Could you check a few things on this drawing? It's one solid part, dimensions in mm from its lowest x, y, z. Give positions to 0.01 mm unless a question says otherwise; leave off trailing zeros. Order: outer loops, then holes, each group sorted by start corner. A loop starts at its lowest first (then second) coordinate and runs counter-clockwise, first axis right, second up.
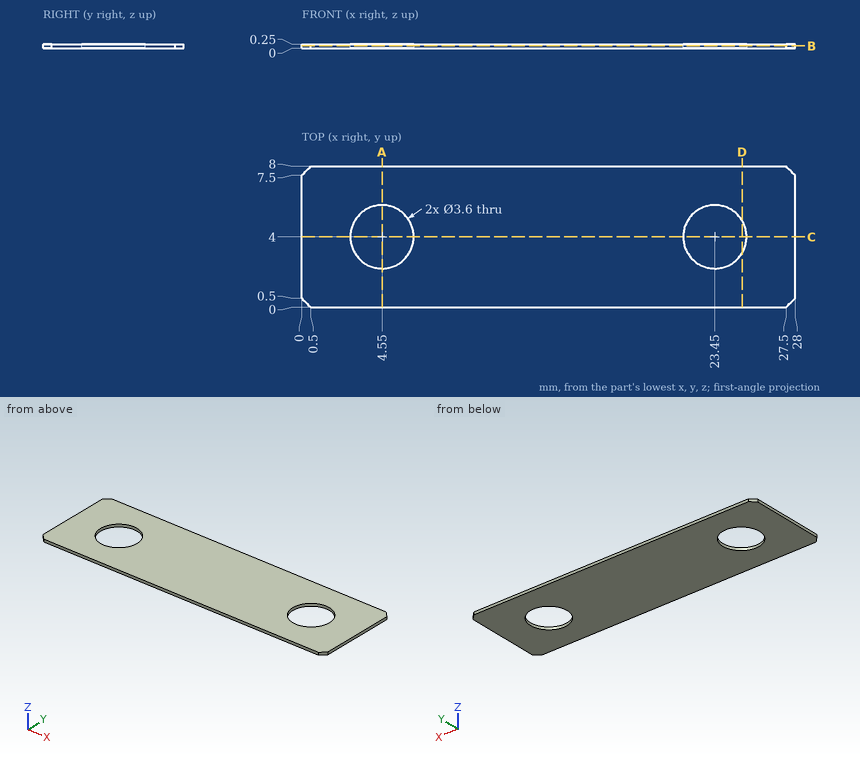
Item 1: Imagine slicing it at B-B on z = 0.15. List the corners of the cut face in (x, y) for me.
Findings:
outline: (0, 0.5) - (0.5, 0) - (27.5, 0) - (28, 0.5) - (28, 7.5) - (27.5, 8) - (0.5, 8) - (0, 7.5) - close; hole circle Ø3.6 at (4.55, 4); hole circle Ø3.6 at (23.45, 4)
Item 2: Imagine slicing it at A-A on x = 4.55. List the corners of the cut face in (y, z) for me.
Findings:
outline: (0, 0) - (2.2, 0) - (2.2, 0.25) - (0, 0.25) - close; (5.8, 0) - (8, 0) - (8, 0.25) - (5.8, 0.25) - close
Item 3: Imagine slicing it at C-C on y = 4. List the corners of the cut face in (x, z) for me.
Findings:
outline: (0, 0) - (2.75, 0) - (2.75, 0.25) - (0, 0.25) - close; (6.35, 0) - (21.65, 0) - (21.65, 0.25) - (6.35, 0.25) - close; (25.25, 0) - (28, 0) - (28, 0.25) - (25.25, 0.25) - close
Item 4: Please list where these lines run through material, in increasing order: line 1 along Y through (x, z) = (23.45, 0.1); line 2 along X through (y, z) = (4.25, 0.15); line 3 along X through (y, z) = (2.5, 0.15).
Findings:
line 1: y = 0 to 2.2, 5.8 to 8
line 2: x = 0 to 2.77, 6.33 to 21.67, 25.23 to 28
line 3: x = 0 to 3.56, 5.54 to 22.46, 24.44 to 28
Item 5: Imagine slicing it at D-D on x = 25. List the corners of the cut face in (y, z) for me.
Findings:
outline: (0, 0) - (3.08, 0) - (3.08, 0.25) - (0, 0.25) - close; (4.92, 0) - (8, 0) - (8, 0.25) - (4.92, 0.25) - close
